Geometry: see drawing. Coordinates: mm, zero at the bounding-box minimum. Give positions to 0.01 mm unless a question says otherwise; leave off trailing zeros. Loops run counter-clockwise (first coordinate to the right, second up) from the corner with the lowest first, then second, coordinate; pieces in that order, holes last. Notation, with made-up numbers: (60, 19) -> (90, 19) arc R17 ccw to (90, 24) -> close; hole circle Ø10 at (-31, 72.5). An arc over 180 degrees is marked (long way). Answer in a Markdown table with one row per item. Add a question column.
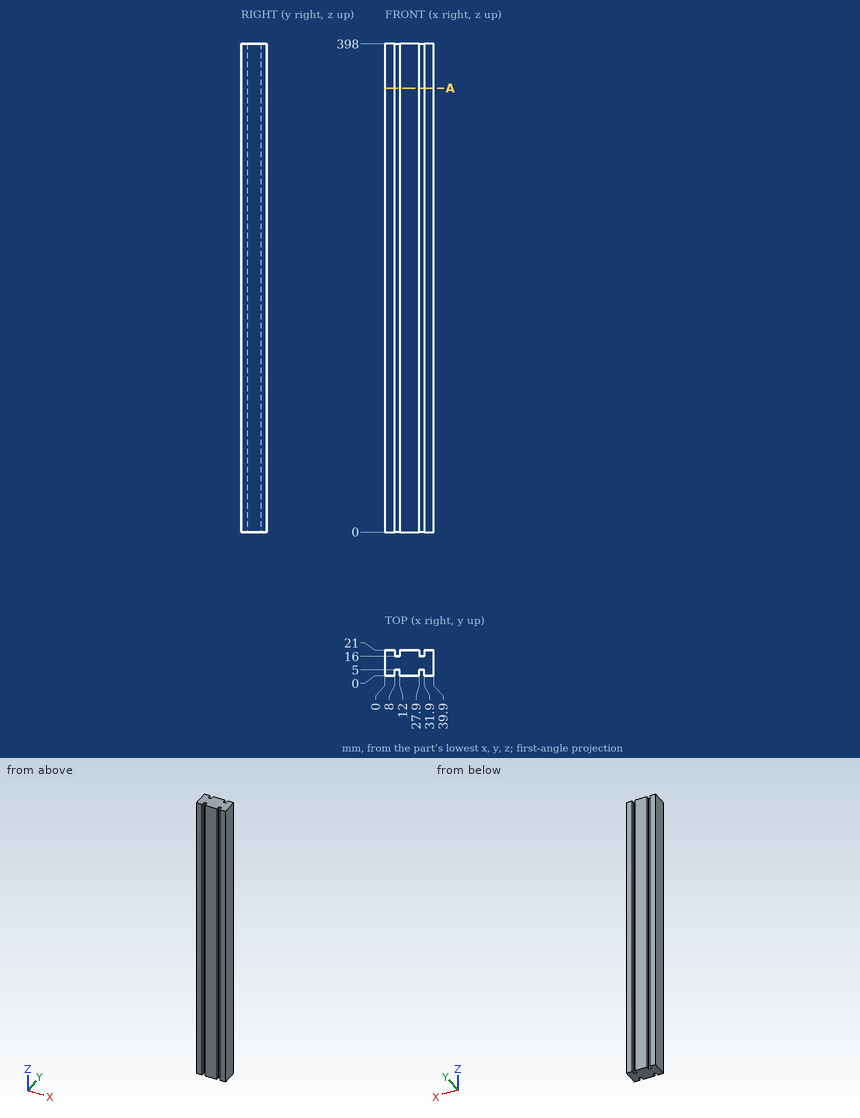
1) Section A-A on z = 362. Output: boundary loops of the cut face in (x, y), and give its area (3 significant figures).
2) Material intervals for line 1 along X through (y, z) = (1, 54.5); line 2 along Y through (x, z) = (31.5, 220), sorted ascending.
3) Pin query (flat end, axial travel): pin 1 (2 mm diameter, centred on x = 29.5, z = 112.5, fed in from +Y); pin 2 (2 mm diameter, centred on x = 30.5, z = 202.5, fed in from -Y). Return the tip coordinate at first contact, or that it passes through.
Working result:
| question | item | result |
|---|---|---|
| 1 | outline | (0, 0) -> (8, 0) -> (8, 5) -> (12, 5) -> (12, 0) -> (27.9, 0) -> (27.9, 5) -> (31.9, 5) -> (31.9, 0) -> (39.9, 0) -> (39.9, 21) -> (31.9, 21) -> (31.9, 16) -> (27.9, 16) -> (27.9, 21) -> (12, 21) -> (12, 16) -> (8, 16) -> (8, 21) -> (0, 21) -> close |
| 1 | area | 758 mm2 |
| 2 | line 1 | x = 0 to 8, 12 to 27.9, 31.9 to 39.9 |
| 2 | line 2 | y = 5 to 16 |
| 3 | pin 1 | stops at y = 16 |
| 3 | pin 2 | stops at y = 5 |
